Work out the finished part from the listing and answer in its coordinate system (mm). A direction names the side the tool comes from. Round coordinates to 2 decimals unless told otherwise and drop trailing zeros. Write each loop counter-clockwise with the first axis right and the second up, starting at its lowest first coordinate (ties: lowest second). Pieces come first, ordered by that corner, then holes. Notation, with made-up numbers: M 72.5,56 L 125.5,56 A24 ccw 125.5,88 Z; hole C 60,-25 d7. An arc over 180 degrees is marked long. One line per item, written item: value. Start each with the question number.
Q1. Find section D-D (x = 10). Write down the section's boundary in (y, z), and give its area (3 significant figures).
Q2. Find section C-C (z = 5). Write down the section's boundary in (x, y), and give its area (3 significant figures).
Q3. The mould has two halves that part along X. Classify faces 4 (the flat face through (45, 10, 6)), 5 (the flat face through (16, 16, 15)), 6 (the cylindrical face through (44.985, 29.34, 39.213)): released by +X, released by -X, zero draft, split by the parting line, or undercut.
Q4. Find section B-B (x = 30). Write down the section's boundary in (y, z).
Q5. A tool of negligible diameter and unlimited length cuts with its end or side. For faces 1 (the flat face through (35, 43, 50)), 2 (the cylindrical face through (43.31, 10.29, 10.56)), 3 (the flat face through (0, 30, 8)), from which of +Z, -Z, +X, -X, +Y, -Y can it reach the whole face along a straight path? Write none if from no direction.
Q6. Given pin 1 Ø3.5 at (x, y) = (31, 43.5) entering from -Z; pin 2 Ø1.1 at (y, z) = (43.5, 49.5) entering from +X; pin 3 Ø0.6 at (y, z) = (17, 49) entering from -X; pin 4 Ø4 at (x, y) = (6.5, 9.5) entering from +Z, each flat-ended and moving along its own axis, determine where each tip first touches the part or whether it passes through.
Q7. Consider probe 1 along X at (y, z) = (5, 7.5); probe 2 along Y at (x, z) = (6.5, 14.5); probe 3 along X at (y, z) = (35, 56). Determine where each line is inside the solid, lowest interval first.
Q8. Find section A-A (y = 10). Write down the section's boundary in (x, z), and give its area (3 significant figures).
from build123d import *

# Parameters (mm, degrees)
ESBO_O1_W                = 60
ESBO_O1_H                = 15
RESSALTO_EXTRUS_O1_DEPTH = 60
ESBO_O4_R                = 6.5
CORTE_EXTRUS_O1_DEPTH    = 9
ESBO_O5_R                = 4.5
CORTE_EXTRUS_O2_DEPTH    = 6
ESBO_O6_R                = 15
RESSALTO_EXTRUS_O3_DEPTH = 45
ESBO_O7_R                = 13
CORTE_EXTRUS_O3_DEPTH    = 104.923048454
FILETE2_R                = 4
ESBO_O8_R                = 7.5
CORTE_EXTRUS_O10_DEPTH   = 104.923048454
ESBO_O9_W                = 10
ESBO_O9_H                = 10
CORTE_EXTRUS_O11_DEPTH   = 104.923048512
FILETE3_R                = 8


with BuildPart() as part:
    # Esboço1 → Ressalto-extrusão1 (new body)
    with BuildSketch(Plane(origin=(0, 0, 0), x_dir=(1, 0, 0), z_dir=(0, 1, 0))):
        with Locations((30, -7.5)):
            Rectangle(ESBO_O1_W, ESBO_O1_H)
    extrude(amount=RESSALTO_EXTRUS_O1_DEPTH)

    # Esboço4 → Corte-extrusão1 (cut)
    with BuildSketch(Plane.XY.offset(15)):
        with Locations((9.802292797, 50)):
            Circle(ESBO_O4_R)
        with Locations((49.802292797, 50)):
            Circle(ESBO_O4_R)
        with Locations((9.802292797, 10)):
            Circle(ESBO_O4_R)
        with Locations((49.802292797, 10)):
            Circle(ESBO_O4_R)
    extrude(amount=-CORTE_EXTRUS_O1_DEPTH, mode=Mode.SUBTRACT)

    # Esboço5 → Corte-extrusão2 (cut)
    with BuildSketch(Plane(origin=(0, 0, 0), x_dir=(-1, 0, 0), z_dir=(0, 0, -1))):
        with Locations((-50, 50)):
            Circle(ESBO_O5_R)
        with Locations((-10, 50)):
            Circle(ESBO_O5_R)
        with Locations((-50, 10)):
            Circle(ESBO_O5_R)
        with Locations((-10, 10)):
            Circle(ESBO_O5_R)
    extrude(amount=-CORTE_EXTRUS_O2_DEPTH, mode=Mode.SUBTRACT)

    # Esboço6 → Ressalto-extrusão3 (add)
    with BuildSketch(Plane.XY.offset(15)):
        with Locations(Location((30, 30, 0), (0, 0, 180))):
            Circle(ESBO_O6_R)
    extrude(amount=RESSALTO_EXTRUS_O3_DEPTH)

    # Esboço7 → Corte-extrusão3 (cut, through all)
    with BuildSketch(Plane.XY.offset(60)):
        with Locations((30, 30)):
            Circle(ESBO_O7_R)
    extrude(amount=-CORTE_EXTRUS_O3_DEPTH, mode=Mode.SUBTRACT)

    # Filete2
    filete2_edges = [part.edges().sort_by_distance(p)[0] for p in [
        (45, 30, 15),
    ]]
    fillet(filete2_edges, radius=FILETE2_R)

    # Esboço8 → Corte-extrusão10 (cut, through all)
    with BuildSketch(Plane(origin=(0, 0, 0), x_dir=(0, 0, -1), z_dir=(1, 0, 0))):
        with Locations(Location((-30, 30, 0), (0, 0, 180))):
            Circle(ESBO_O8_R)
    extrude(amount=CORTE_EXTRUS_O10_DEPTH, mode=Mode.SUBTRACT)

    # Esboço9 → Corte-extrusão11 (cut, through all)
    with BuildSketch(Plane(origin=(0, 0, 0), x_dir=(1, 0, 0), z_dir=(0, 1, 0))):
        with Locations((30, -50)):
            Rectangle(ESBO_O9_W, ESBO_O9_H)
    extrude(amount=CORTE_EXTRUS_O11_DEPTH, mode=Mode.SUBTRACT)

    # Filete3
    filete3_edges = [part.edges().sort_by_distance(p)[0] for p in [
        (60, 60, 7.5),
        (60, 0, 7.5),
        (0, 0, 7.5),
        (0, 60, 7.5),
    ]]
    fillet(filete3_edges, radius=FILETE3_R)


solid = part.part
The answers:
1. outline: M 0,0 L 5.5,0 L 5.5,6 L 3.5,6 L 3.5,15 L 0,15 Z; M 14.5,0 L 45.5,0 L 45.5,6 L 43.5,6 L 43.5,15 L 16.5,15 L 16.5,6 L 14.5,6 Z; M 54.5,0 L 60,0 L 60,15 L 56.5,15 L 56.5,6 L 54.5,6 Z
1. area: 558 mm2
2. outline: M 0,8 A8 ccw 8,0 L 52,0 A8 ccw 60,8 L 60,52 A8 ccw 52,60 L 8,60 A8 ccw 0,52 Z; hole C 10,10 d9; hole C 10,50 d9; hole C 30,30 d26; hole C 50,10 d9; hole C 50,50 d9
2. area: 2,760 mm2
3. face 4: undercut
3. face 5: zero draft
3. face 6: split by the parting line
4. outline: M 0,0 L 17,0 L 17,45 L 15,45 L 15,19 A4 cw 11,15 L 0,15 Z; M 15,55 L 17,55 L 17,60 L 15,60 Z; M 43,0 L 60,0 L 60,15 L 49,15 A4 cw 45,19 L 45,45 L 43,45 Z; M 43,55 L 45,55 L 45,60 L 43,60 Z
5. face 1: +Y, -Y
5. face 2: +Z
5. face 3: +Z, -Z, -X, +Y, -Y
6. pin 1: z = 0
6. pin 2: x = 37.57
6. pin 3: x = 22.02
6. pin 4: z = 6
7. probe 1: 0.58 to 5.65, 13.96 to 45.65, 53.96 to 59.42
7. probe 2: 0.14 to 4.4, 15.6 to 44.4, 55.6 to 59.86
7. probe 3: 15.86 to 18, 42 to 44.14
8. outline: M 0,0 L 5.5,0 L 5.5,6 L 3.3,6 L 3.3,15 L 0,15 Z; M 14.5,0 L 45.5,0 L 45.5,6 L 43.3,6 L 43.3,15 L 16.3,15 L 16.3,6 L 14.5,6 Z; M 54.5,0 L 60,0 L 60,15 L 56.3,15 L 56.3,6 L 54.5,6 Z
8. area: 558 mm2
